```python
from build123d import *

# Parameters (mm, degrees)
SKETCH1_W                      = 330.2
SKETCH1_H                      = 228.6
BASE_PLATE_DEPTH               = 6.35
SLOTS_DEPTH                    = 7.35
FEET_CONNECTION_HOLE_D         = 8.7376
F_1_4_0_25_DIAMETER_HOLE1_D    = 6.35
F_5_16_0_3125_DIAMETER_HOLE1_D = 7.9375
ESD_CONNECTION_HOLE_D          = 4.7625


with BuildPart() as part:
    # Sketch1 → base plate (new body)
    with BuildSketch(Plane(origin=(0, 0, 0), x_dir=(1, 0, 0), z_dir=(0, 1, 0))):
        with Locations((165.1, -114.3)):
            Rectangle(SKETCH1_W, SKETCH1_H)
    extrude(amount=-BASE_PLATE_DEPTH)

    # Sketch3 → slots (cut, through all)
    with BuildSketch(Plane(origin=(0, 0, 0), x_dir=(1, 0, 0), z_dir=(0, 1, 0))):
        with BuildLine():
            ThreePointArc((37.882935507, -47.754508291), (37.882935507, -50.582935507), (35.054508291, -50.582935507))
            Line((35.054508291, -50.582935507), (29.666354619, -45.194781834))
            ThreePointArc((29.666354619, -45.194781834), (29.666354619, -42.366354619), (32.494781834, -42.366354619))
            Line((32.494781834, -42.366354619), (37.882935507, -47.754508291))
        make_face()
        with BuildLine():
            Line((297.705218166, -42.366354619), (292.317064493, -47.754508291))
            ThreePointArc((292.317064493, -47.754508291), (292.317064493, -50.582935507), (295.145491709, -50.582935507))
            Line((295.145491709, -50.582935507), (300.533645381, -45.194781834))
            ThreePointArc((300.533645381, -45.194781834), (300.533645381, -42.366354619), (297.705218166, -42.366354619))
        make_face()
        with BuildLine():
            Line((283.336808372, -62.391618843), (288.724962045, -57.00346517))
            ThreePointArc((288.724962045, -57.00346517), (288.724962045, -54.175037955), (285.89653483, -54.175037955))
            Line((285.89653483, -54.175037955), (280.508381157, -59.563191628))
            ThreePointArc((280.508381157, -59.563191628), (280.508381157, -62.391618843), (283.336808372, -62.391618843))
        make_face()
        with BuildLine():
            ThreePointArc((288.724962045, -171.59653483), (288.724962045, -174.424962045), (285.89653483, -174.424962045))
            Line((285.89653483, -174.424962045), (280.508381157, -169.036808372))
            ThreePointArc((280.508381157, -169.036808372), (280.508381157, -166.208381157), (283.336808372, -166.208381157))
            Line((283.336808372, -166.208381157), (288.724962045, -171.59653483))
        make_face()
        with BuildLine():
            ThreePointArc((292.317064493, -180.845491709), (292.317064493, -178.017064493), (295.145491709, -178.017064493))
            Line((295.145491709, -178.017064493), (300.533645381, -183.405218166))
            ThreePointArc((300.533645381, -183.405218166), (300.533645381, -186.233645381), (297.705218166, -186.233645381))
            Line((297.705218166, -186.233645381), (292.317064493, -180.845491709))
        make_face()
        with BuildLine():
            Line((32.494781834, -186.233645381), (37.882935507, -180.845491709))
            ThreePointArc((37.882935507, -180.845491709), (37.882935507, -178.017064493), (35.054508291, -178.017064493))
            Line((35.054508291, -178.017064493), (29.666354619, -183.405218166))
            ThreePointArc((29.666354619, -183.405218166), (29.666354619, -186.233645381), (32.494781834, -186.233645381))
        make_face()
        with BuildLine():
            Line((46.863191628, -166.208381157), (41.475037955, -171.59653483))
            ThreePointArc((41.475037955, -171.59653483), (41.475037955, -174.424962045), (44.30346517, -174.424962045))
            Line((44.30346517, -174.424962045), (49.691618843, -169.036808372))
            ThreePointArc((49.691618843, -169.036808372), (49.691618843, -166.208381157), (46.863191628, -166.208381157))
        make_face()
        with BuildLine():
            Line((46.863191628, -62.391618843), (41.475037955, -57.00346517))
            ThreePointArc((41.475037955, -57.00346517), (41.475037955, -54.175037955), (44.30346517, -54.175037955))
            Line((44.30346517, -54.175037955), (49.691618843, -59.563191628))
            ThreePointArc((49.691618843, -59.563191628), (49.691618843, -62.391618843), (46.863191628, -62.391618843))
        make_face()
    extrude(amount=-SLOTS_DEPTH, mode=Mode.SUBTRACT)

    # Feet connection hole (through all)
    with Locations(Plane(origin=(0, 0, 0), x_dir=(1, 0, 0), z_dir=(0, 1, 0))):
        with Locations((12.7, -215.9), (317.5, -12.7), (317.5, -215.9), (12.7, -12.7)):
            Hole(FEET_CONNECTION_HOLE_D / 2)

    # 1/4 (0.25) Diameter Hole1 (through all)
    with Locations(Plane(origin=(0, 0, 0), x_dir=(1, 0, 0), z_dir=(0, 1, 0))):
        with Locations((28.575, -207.01), (301.625, -207.01)):
            Hole(F_1_4_0_25_DIAMETER_HOLE1_D / 2)

    # 5/16 (0.3125) Diameter Hole1 (through all)
    with Locations(Plane(origin=(0, 0, 0), x_dir=(1, 0, 0), z_dir=(0, 1, 0))):
        with Locations((41.275, -35.56), (288.925, -35.56)):
            Hole(F_5_16_0_3125_DIAMETER_HOLE1_D / 2)

    # ESD Connection hole (through all)
    with Locations(Plane(origin=(0, 0, 0), x_dir=(1, 0, 0), z_dir=(0, 1, 0))):
        with Locations((165.1, -15.24), (164.768662044, -213.266978445)):
            Hole(ESD_CONNECTION_HOLE_D / 2)


solid = part.part
```
Can you work these out from the model? Positions are in its coordinate system, mm. Coordinates: 2 decimals unless noted, no trailing zeros. Write each loop counter-clockwise with the first axis right and the second up, starting at its lowest first coordinate (ties: lowest second). Pieces come first, ordered by that corner, then holes. Notation, with made-up numbers: (25, 34.25) - (58, 34.25) arc R15 cw to (58, 53.25) - close; hole circle Ø2 at (83.5, 79). An arc over 180 degrees is marked (long way). Return JSON: item names as keys, results as strings.
Q1. I'm going to push a flat-ended pin straight in: pin 1 Ø8 at (x, z) = (317.5, 12.7) entering from -Y. Where does the tip first touch, or does it pass through?
Computed values:
{"pin 1": "passes through"}
Q2. Please list where these lines run through material, in increasing order: L1, parallel to Z at x = 165.1, y = -3.75; L2, parallel to Z at x = 12.7, y = -2.5; L3, parallel to X at y = -4.25, z = 206.5. Write a range as from..to.
Computed values:
{"L1": "z = 0..12.86, 17.62..210.91, 215.63..228.6", "L2": "z = 0..8.33, 17.07..211.53, 220.27..228.6", "L3": "x = 0..25.44, 31.71..298.49, 304.76..330.2"}
Q3. If we section it at A-A (x = 12.7): Please give me the cut outline in (y, z), then the cut area to 3 significant figures.
Computed values:
{"outline": "(-6.35, 0) - (0, 0) - (0, 8.33) - (-6.35, 8.33) - close; (-6.35, 17.07) - (0, 17.07) - (0, 211.53) - (-6.35, 211.53) - close; (-6.35, 220.27) - (0, 220.27) - (0, 228.6) - (-6.35, 228.6) - close", "area": "1,340 mm2"}
Q4. Thinking about a two-plate mould opening in X: for faces 1 (the flat face through (163, -6.35, 113)), 2 (the flat face through (0, -3, 116)), 3 (the cylindrical face through (29.3, -3.2, 210.1)), which applies, +X half, -X half, draft (parallel to the pull), parting line (faces both ways), or undercut?
Computed values:
{"face 1": "draft", "face 2": "-X half", "face 3": "undercut"}
